Could you check a few things on this model? Use its own coordinates, in mm. A direction names the side the tool comes from. Give positions to 0.01 mm unless a question says otherwise; leave off trailing zeros. Write each loop counter-clockwise with the first axis right and the second up, starting at its lowest first coordinate (ties: lowest second). Pieces come first, ordered by that corner, then holes. Notation, with made-up numbers: M 27,85 L 38,85 A22 ccw 38,103 Z; hole C -33.5,-23 d3. An arc over 180 degrees is marked long. One line per item, written item: value.
```python
from build123d import *
from build123d.topology import SkipClean

# Parameters (mm, degrees)
SKETCH2_R           = 14
BOSS_EXTRUDE2_DEPTH = 19
SKETCH3_R           = 4.5
BOSS_EXTRUDE3_DEPTH = 1.5
SKETCH4_R           = 2.5
BOSS_EXTRUDE4_DEPTH = 2.5
SKETCH5_R           = 2
BOSS_EXTRUDE5_DEPTH = 1
SKETCH6_W           = 14.6
SKETCH6_H           = 9.231468238
BOSS_EXTRUDE6_DEPTH = 17
BOSS_EXTRUDE7_DEPTH = 6


with BuildPart() as part:
    # Sketch2 → Boss-Extrude2 (new body)
    with BuildSketch(Plane.XY):
        Circle(SKETCH2_R)
    extrude(amount=BOSS_EXTRUDE2_DEPTH)

    # Sketch3 → Boss-Extrude3 (add)
    with BuildSketch(Plane.XY.offset(19)):
        with Locations((0, 8)):
            Circle(SKETCH3_R)
    extrude(amount=BOSS_EXTRUDE3_DEPTH)

    # Sketch4 → Boss-Extrude4 (add)
    with BuildSketch(Plane.XY.offset(20.5)):
        with Locations((0, 8)):
            Circle(SKETCH4_R)
    extrude(amount=BOSS_EXTRUDE4_DEPTH)

    # Sketch5 → Boss-Extrude5 (add)
    with BuildSketch(Plane.XY.offset(19)):
        with BuildLine():
            ThreePointArc((17.5, -3.5), (21, 0), (17.5, 3.5))
            Line((17.5, 3.5), (13.555441712, 3.5))
            ThreePointArc((13.555441712, 3.5), (13.888415748, 1.764060095), (14, 0))
            ThreePointArc((14, 0), (13.888415748, -1.764060095), (13.555441712, -3.5))
            Line((13.555441712, -3.5), (17.5, -3.5))
        make_face()
        with Locations((17.5, 0)):
            Circle(SKETCH5_R, mode=Mode.SUBTRACT)
        with BuildLine():
            ThreePointArc((-13.555441712, -3.5), (-14, 0), (-13.555441712, 3.5))
            Line((-13.555441712, 3.5), (-17.5, 3.5))
            ThreePointArc((-17.5, 3.5), (-21, 0), (-17.5, -3.5))
            Line((-17.5, -3.5), (-13.555441712, -3.5))
        make_face()
        with Locations((-17.5, 0)):
            Circle(SKETCH5_R, mode=Mode.SUBTRACT)
    extrude(amount=-BOSS_EXTRUDE5_DEPTH)

    # Sketch6 → Boss-Extrude6 (add)
    with BuildSketch(Plane.XY.offset(19)):
        with Locations((0, -12.384265881)):
            Rectangle(SKETCH6_W, SKETCH6_H)
    extrude(amount=-BOSS_EXTRUDE6_DEPTH)

    # Sketch7 → Boss-Extrude7 (add)
    with SkipClean():  # the faces are left unmerged after this step: merging them gives an invalid solid
        with BuildSketch(Plane.XY.offset(23)):
            with BuildLine():
                Line((-1.5, 6), (-1.5, 10))
                ThreePointArc((-1.5, 10), (0, 10.5), (1.5, 10))
                Line((1.5, 10), (1.5, 6))
                ThreePointArc((1.5, 6), (0, 5.5), (-1.5, 6))
            make_face()
        extrude(amount=BOSS_EXTRUDE7_DEPTH)


solid = part.part
```
1) On a 3-axis mill with a long thin cutter (end or side, diameter ignored), from which of +Z, -Z, +X, -X, +Y, -Y can I reach the whole of each face in a straight line? I mean faces 4 (the face through (15.6, 3.5, 18.5)), 5 (the face through (-0.59, 12.46, 19.74)), 6 (the face through (-15.6, -3.5, 18.5)), 7 (the face through (-15.5, 3.5, 18.5)). Say none if no direction works.
Outcome:
face 4: +Z, -Z, +X, +Y
face 5: +Z
face 6: +Z, -Z, -X, -Y
face 7: +Z, -Z, -X, +Y
2) If we section it at B-B, the plane x = 0: Write out the boundary of the cut face in (y, z).
Outcome:
outline: M -17,2 L -14,2 L -14,0 L 14,0 L 14,19 L 12.5,19 L 12.5,20.5 L 10.5,20.5 L 10.5,29 L 5.5,29 L 5.5,20.5 L 3.5,20.5 L 3.5,19 L -17,19 Z
3) If we section it at D-D, the plane y = 8: Write out the boundary of the cut face in (x, z), then the cut area to 3 significant figures.
Outcome:
outline: M -11.49,0 L 11.49,0 L 11.49,19 L 4.5,19 L 4.5,20.5 L 2.5,20.5 L 2.5,23 L 1.5,23 L 1.5,29 L -1.5,29 L -1.5,23 L -2.5,23 L -2.5,20.5 L -4.5,20.5 L -4.5,19 L -11.49,19 Z
area: 481 mm^2
4) We'd pull the mould along X, two halves only. Please class faces 1 (the face through (7.3, -15, 11)), 2 (the face through (15.9, -1.2, 18.5)), 3 (the face through (2, 6, 20.5)): pulls with the +X half, pulls with the -X half, needs draft (parallel to the pull), parting line crosses it, or undercut.
Outcome:
face 1: pulls with the +X half
face 2: undercut
face 3: needs draft
5) If we section it at C-C, the plane z = 9: Write out the boundary of the cut face in (x, y), then the cut area to 3 significant figures.
Outcome:
outline: M -7.3,-17 L 7.3,-17 L 7.3,-11.95 A14 ccw long -7.3,-11.95 Z
area: 669 mm^2
6) If we section it at A-A, the plane y = 0: Write out the boundary of the cut face in (x, z), then the cut area to 3 significant figures.
Outcome:
outline: M -21,18 L -19.5,18 L -19.5,19 L -21,19 Z; M -15.5,18 L -14,18 L -14,0 L 14,0 L 14,18 L 15.5,18 L 15.5,19 L -15.5,19 Z; M 19.5,18 L 21,18 L 21,19 L 19.5,19 Z
area: 538 mm^2
7) I'm going to push flat-ended pins straight in: pin 1 (8 mm diameter, centred on y = 7.5, z = 8, fed in from -X); pin 2 (12 mm diameter, centred on y = 10.5, z = 3, fed in from -X); pin 3 (3.5 mm diameter, centred on x = 16.5, y = 1, fed in from -Z). Where does each tip first touch, or does it pass through?
Outcome:
pin 1: stops at x = -13.56
pin 2: stops at x = -13.26
pin 3: stops at z = 18
8) Please list where these lines run through material, in increasing order: L1, parallel to Y at x = 17.5, z = 18.6; L2, parallel to Z at x = -0.5, y = 0; L3, parallel to X at y = -14, z = 5.75. Write a range as from..to.
Outcome:
L1: y = -3.5..-2, 2..3.5
L2: z = 0..19
L3: x = -7.3..7.3
